Input: dimensioned drawing with shaded views. Units: mm. Origin: part minimum x, y, z. A direction names the side the tool comes from. Round coordinates to 2 decimals unless told otherwise and drop trailing zeros. Write each loop counter-clockwise with the first axis right and the second up, starting at its lowest first coordinate (ties: lowest second). Pieces come first, ordered by that corner, then holes. Notation, with made-up numbers: (83.25, -17.75) -> (112.25, -17.75) arc R8 cw to (112.25, -11.75) -> close; hole circle Ø11 at (42, -28.75). An arc over 180 degrees is marked (long way). Return JSON: item names as keys, results as strings. Group by question number.
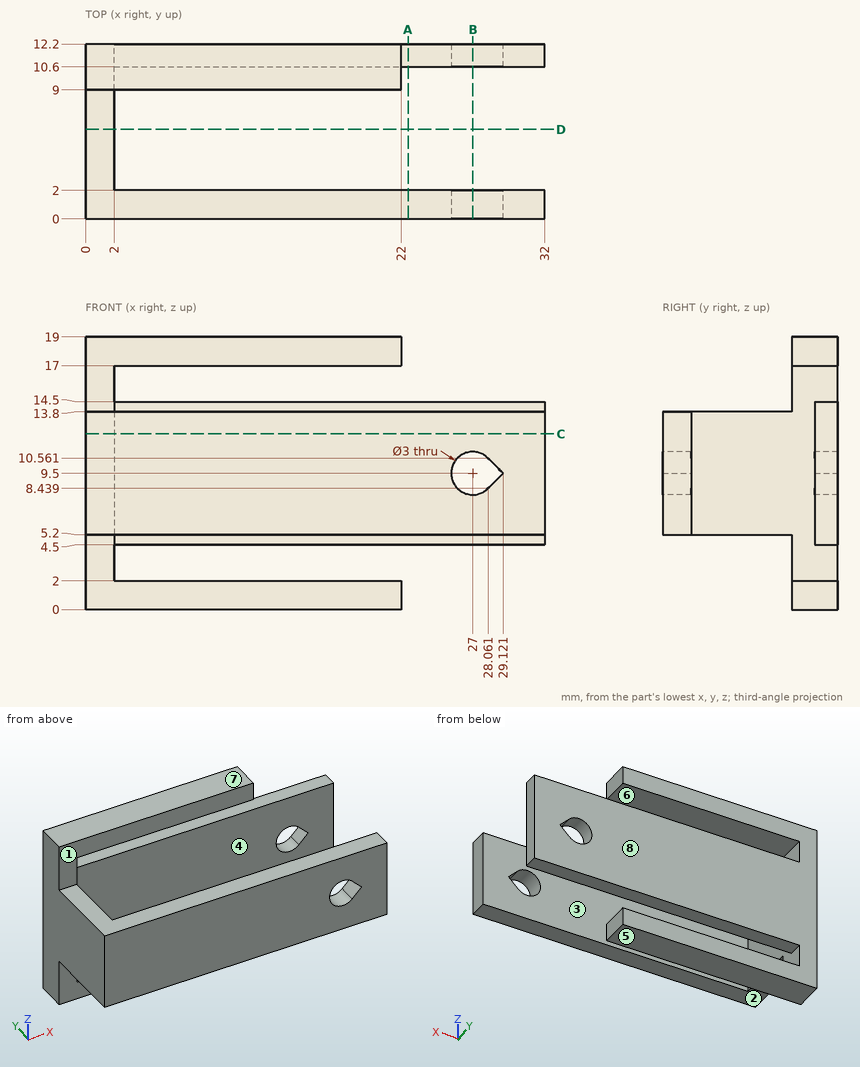
Item 1: Pull-direction query (Z, two-part tool) for the marked faces 5, 6, 7 and 8; classes: +Z half, -Z half, draft (parallel to the pull), parting line (faces both ways), or undercut.
Item 2: Cut plane A-A on x = 22.5. Output: boundary loops of the cut face in (y, z).
Item 3: Cut plane B-B on x = 27. Output: boundary loops of the cut face in (y, z), and give its area (3 significant figures).
Item 4: Cut plane C-C on z = 12.25. Output: boundary loops of the cut face in (x, y).
Item 5: Cut plane D-D on y = 6.25. Output: boundary loops of the cut face in (x, z).
Item 6: First-contact query: pin 1 Ø1.6 at (x, z) = (16, 17.5) entering from -Y; pin 2 Ø2 at (y, z) = (10.5, 18) entering from +X; pin 3 Ø4.5 at (x, y) = (13.5, 3.5) entering from +Z; pin 4 Ø2.5 at (x, z) = (27, 9.5) entering from -Y. Flat tips, straight axial feed; report the tip coordinate or a pass-through.
Item 7: Material intervals for probe 1 along Z at (x, y) = (15, 11.25); probe 2 along Y at (x, z) = (7.5, 6.75); probe 3 along Z at (x, y) = (27, 1.6), sorted ascending.
Item 8: Set-up query: the marked faces 1, 2, 3 and 4. Return all of +Z, -Z, +X, -X, +Y, -Y with unobstructed straight access to the full face (end or side cutting, diameter ignored); none if empty.
Here are the results:
{
 "1": {"face 5": "-Z half", "face 6": "undercut", "face 7": "+Z half", "face 8": "draft"},
 "2": {"outline": "(0, 5.2) -> (2, 5.2) -> (2, 13.8) -> (0, 13.8) -> close; (10.6, 4.5) -> (12.2, 4.5) -> (12.2, 14.5) -> (10.6, 14.5) -> close"},
 "3": {"outline": "(0, 5.2) -> (2, 5.2) -> (2, 8) -> (0, 8) -> close; (0, 11) -> (2, 11) -> (2, 13.8) -> (0, 13.8) -> close; (10.6, 4.5) -> (12.2, 4.5) -> (12.2, 8) -> (10.6, 8) -> close; (10.6, 11) -> (12.2, 11) -> (12.2, 14.5) -> (10.6, 14.5) -> close", "area": "22.4 mm^2"},
 "4": {"outline": "(0, 0) -> (32, 0) -> (32, 2) -> (2, 2) -> (2, 10.6) -> (32, 10.6) -> (32, 12.2) -> (0, 12.2) -> close"},
 "5": {"outline": "(0, 5.2) -> (2, 5.2) -> (2, 13.8) -> (0, 13.8) -> close"},
 "6": {"pin 1": "stops at y = 9", "pin 2": "stops at x = 22", "pin 3": "stops at z = 13.8", "pin 4": "passes through"},
 "7": {"probe 1": "z = 0 to 2, 4.5 to 14.5, 17 to 19", "probe 2": "y = 0 to 2, 10.6 to 12.2", "probe 3": "z = 5.2 to 8, 11 to 13.8"},
 "8": {"face 1": "+Z, +X, -X, -Y", "face 2": "-Z, +X, -X, -Y", "face 3": "+Z, -Z, +X", "face 4": "+X"}
}
